Source: CAD feature listing. Evaluate the final solid. Frame: model axes, mm. A direction names the side the tool comes from. Coordinates: 2 decimals unless noted, no trailing zeros. Write each loop counter-clockwise with the first axis right and the second up, starting at its lowest first coordinate (ties: lowest second). Pieces come first, ordered by that corner, then holes. Notation, with made-up numbers: M 62.5,55 L 74.5,55 A15 ccw 74.5,75 Z; hole C -30.5,8 d6. An arc over 180 degrees is marked long. One line per item, written item: value. Start each with the question number.
Item 1: Cut plane C-C, the plane y = 15.75. Output: boundary loops of the cut face in (x, z), then the cut area to 3 significant figures.
Item 2: Pin query (flat end, axial travel): P1, Ø1, axis at x = -23.5, z = -15.5, coming from the +Y side (3 decimals); P2, Ø1, axis at y = 0.5, z = 73, coming from the -X side; P3, Ø5, axis at y = 18.5, z = -23, coming from the -X side. Return the tip coordinate at first contact, or that it passes through.
Item 3: Cut plane D-D, the plane z = -48. Output: boundary loops of the cut face in (x, y) (3 decimals).
Item 4: Cut plane B-B, the plane x = 0. Output: boundary loops of the cut face in (y, z) (3 decimals), then the cut area to 3 significant figures.
Item 5: Mould query, pull axis Z, two halves, no side actions, for faces 1 (the flat face through (5, 22.225, 12)), 2 (the cylindrical face through (2.75, 9.7, -12.4)), 3 (the cylindrical face through (-22.025, -0.044, -99.184)). Classes: released by +Z, released by -Z, zero draft, split by the parting line, or undercut.
Item 6: Ray query, L1, parallel to Z at x = 0, y = 8.25; L2, parallel to Y at x = -22, z = -23.5 (3 decimals); L3, parallel to X at y = 1, z = -4. Return the intervals inside material, ascending. Write a range as from..to.
Item 7: Cut plane A-A, the plane z = 0. Output: boundary loops of the cut face in (x, y) (3 decimals), then the cut area to 3 significant figures.
Item 8: Set-up query: faces 4 (the flat face through (21, 3.175, -21)), 5 (the flat face through (21, -3.175, 1)). Return all of +Z, -Z, +X, -X, +Y, -Y with unobstructed straight access to the full face (end or side cutting, diameter ignored); none if empty.
```python
from build123d import *

# Parameters (mm, degrees)
F0_R     = 101.6
F1_DEPTH = 3.175
F2_R     = 25.4
F3_DEPTH = 25.4
F4_R     = 12.7
F5_DEPTH = 63.5


with BuildPart() as f1:
    # F0 (on Front) → F1 (new body, symmetric)
    with BuildSketch(Plane.XZ):
        Circle(F0_R)
    extrude(amount=F1_DEPTH, both=True)

    # F2 (on face) → F3 (join)
    with BuildSketch(Plane.XZ.offset(3.175)):
        Circle(F2_R)
    extrude(amount=-F3_DEPTH)

    # F4 (on face) → F5 (cut, symmetric)
    with BuildSketch(Plane(origin=(0, 3.175, 0), x_dir=(-1, 0, 0), z_dir=(0, 1, 0))):
        Circle(F4_R)
    extrude(amount=F5_DEPTH, both=True, mode=Mode.SUBTRACT)


solid = f1.part
```
From the geometry:
1. outline: C 0,0 d50.8; hole C 0,0 d25.4
1. area: 1,520 mm²
2. P1: stops at y = 3.175
2. P2: stops at x = -71.18
2. P3: stops at x = -15
3. outline: M -89.546,-3.175 L 89.546,-3.175 L 89.546,3.175 L -89.546,3.175 Z
4. outline: M -3.175,-101.6 L 3.175,-101.6 L 3.175,-25.4 L 22.225,-25.4 L 22.225,-12.7 L -3.175,-12.7 Z; M -3.175,12.7 L 22.225,12.7 L 22.225,25.4 L 3.175,25.4 L 3.175,101.6 L -3.175,101.6 Z
4. area: 1,610 mm²
5. face 1: zero draft
5. face 2: undercut
5. face 3: split by the parting line
6. L1: z = -25.4..-12.7, 12.7..25.4
6. L2: y = -3.175..3.175
6. L3: x = -101.52..-12.05, 12.05..101.52
7. outline: M -101.6,-3.175 L -12.7,-3.175 L -12.7,22.225 L -25.4,22.225 L -25.4,3.175 L -101.6,3.175 Z; M 12.7,-3.175 L 101.6,-3.175 L 101.6,3.175 L 25.4,3.175 L 25.4,22.225 L 12.7,22.225 Z
7. area: 1,610 mm²
8. face 4: +Y
8. face 5: +Z, -Z, +X, -X, -Y
